Geometry: see drawing. Coordinates: mm, zero at the bounding-box minimum. Round coordinates to 2 decimals unless told otherwise and drop trailing zeros. Loops run counter-clockwise (first coordinate to the right, second up) from the corner with the lowest first, then second, coordinate; pieces in that order, holes last. Notation, with made-up numbers: (-6, -27.75) - (44, -27.75) arc R17 ccw to (44, -4.75) - close; hole circle Ø4 at (80, 21.25). An arc over 180 degrees is marked (long way). Return JSON: item names as keys, results as strings. Group by question number.
1. Section B-B on z = 153. Return loops of the section in (x, y).
2. Section A-A on x = 320. Return loops of the section in (y, z), and give its area (3 significant figures).
3. Material intervals for probe 1 along Z at (x, y) = (180, 17.5); probe 2 along X at (y, z) = (16.75, 250); probe 3 along X at (y, z) = (11.5, 182.5), sorted ascending.
4. First-contact query: pin 1 Ø12 at (y, z) = (7, 143.5) entering from +X; pin 2 Ø7.5 at (x, y) = (368.5, 21) entering from -Z; pin 3 Ø5 at (y, z) = (5.5, 302.5) entering from +X. Flat tips, straight axial feed; report the tip coordinate or a pass-through.
5. Draft query along Z for the marked faces 1, 2 and 3. Return one class per face: +Z half, -Z half, draft (parallel to the pull), parting line (faces both ways), or undercut.
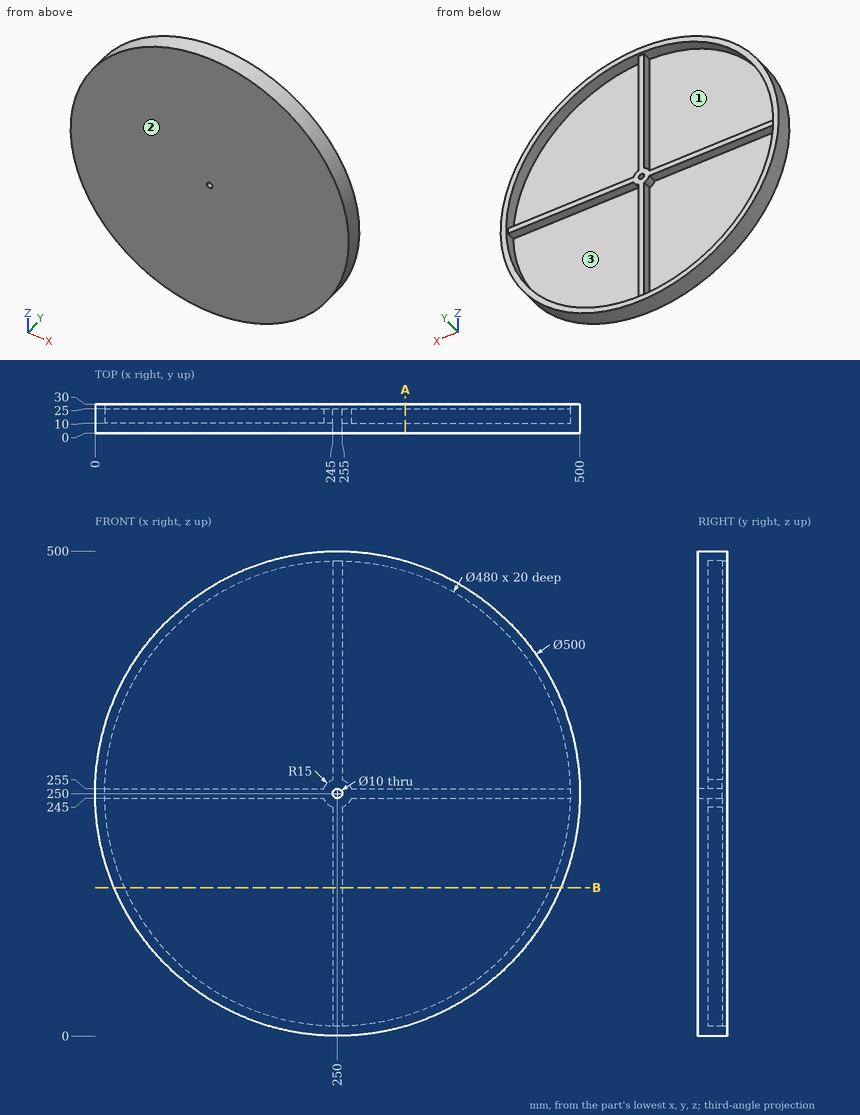
Taken from the geometry:
{
 "1": {"outline": "(19.59, 0) - (480.41, 0) - (480.41, 30) - (469.52, 30) - (469.52, 10) - (255, 10) - (255, 25) - (245, 25) - (245, 10) - (30.48, 10) - (30.48, 30) - (19.59, 30) - close"},
 "2": {"outline": "(0, 10) - (30, 10) - (30, 20.44) - (10, 20.44) - (10, 245) - (25, 245) - (25, 255) - (10, 255) - (10, 479.56) - (30, 479.56) - (30, 490) - (0, 490) - close", "area": "5,370 mm2"},
 "3": {"probe 1": "10 to 20.44, 245 to 255, 479.56 to 490", "probe 2": "0 to 245, 255 to 500", "probe 3": "9.28 to 19.69, 245 to 255, 480.31 to 490.72"},
 "4": {"pin 1": "x = 478.91", "pin 2": "z = 27.89", "pin 3": "x = 494.95"},
 "5": {"face 1": "undercut", "face 2": "draft", "face 3": "undercut"}
}
